The listing builds one solid part. Answer for the finished solid, in the listing's coordinates (mm). A direction names the side the tool comes from. Coordinates: 2 decimals unless noted, no trailing zeros. Loops run counter-clockwise (first coordinate to the right, second up) from the corner with the lowest first, then second, coordinate; pieces in that order, holes last. Notation, with made-up numbers: M 74,-17 L 129,-17 A13 ccw 129,-7 Z; hole C 80,-24 d10. An arc over 180 degrees is marked long. Answer as a JSON object with one key per item and string values. Group by question number.
1. A cutting plane is placed at C-C on x = 0. Give the vertices of the cut face in (y, z).
2. Determine the mould class of faces 5 (the face through (0, -20.32, 19)), 6 (the face through (-38.735, -25, 19)), 7 (the face through (38.011, -21.084, 19.317)) for opening direction X: released by +X, released by -X, zero draft, split by the parting line, or undercut.
3. A cutting plane is placed at A-A on y = 0. Give the vertices of the cut face in (x, z).
4. For faces 1 (the face through (-22.949, -19.556, 19.317)), 2 (the face through (15.875, -16, 19)), 3 (the face through (22.38, -12.44, 19.32)), 4 (the face through (0.132, -24.792, 16.244)), determine the directions among +Z, -Z, +X, -X, +Y, -Y from which every point of the face is accessible in a straight line to the end or side of a thin tool.
5. Given pin 1 (6 mm diameter, centred on x = -31.115, z = 6.35, fed in from +Y); pin 2 (5.5 mm diameter, centred on x = 30.5, z = 19, fed in from +Y); pin 3 (4.5 mm diameter, centred on y = -16, z = 24, fed in from +X); pin 4 (8 mm diameter, centred on y = -15, z = 24, fed in from +X), each flat-ended and moving along its own axis, determine where each tip first touches the part or whether it passes through.
6. Straight lines are drawn through the part: L1, parallel to Z at x = 0, y = -25.65; L2, parallel to X at y = -23, z = 31.75 (3 decimals); L3, parallel to X at y = -22, z = 31.75. For each, find the intervals that lie inside material, in ascending order.
7. A cutting plane is placed at B-B on z = 6.35. State how many separate pieces and enclosed holes the cut face has, and give its area (3 significant figures).
from build123d import *

# Parameters (mm, degrees)
BOSS_EXTRUDE1_DEPTH = 38.1
FILLET1_R           = 6.35
CUT_EXTRUDE1_REACH  = 71.34
SKETCH2_R           = 1.7
SKETCH2_3_R         = 3
SKETCH2_3_R_2       = 1.7
CUT_EXTRUDE2_DEPTH  = 6.35
SKETCH5_W           = 38.1
SKETCH5_H           = 6.35
BOSS_EXTRUDE3_DEPTH = 16.51
SKETCH6_R           = 3.3782
CUT_EXTRUDE3_DEPTH  = 76.254867783
FILLET2_R           = 2.54
BOSS_EXTRUDE4_START = -2.54
SKETCH7_R           = 3
SKETCH7_R_2         = 1.5
BOSS_EXTRUDE4_DEPTH = 2.54


with BuildPart() as part:
    # Sketch1 → Boss-Extrude1 (new body)
    with BuildSketch(Plane.XY):
        with BuildLine():
            Line((22.225, -26.67), (22.225, -12.296722124))
            ThreePointArc((22.225, -12.296722124), (0, 25.4), (-22.225, -12.296722124))
            Line((-22.225, -12.296722124), (-22.225, -26.67))
            Line((-22.225, -26.67), (22.225, -26.67))
        make_face()
        with BuildLine():
            Line((-15.875, -20.32), (15.875, -20.32))
            Line((15.875, -20.32), (15.875, -10.530283709))
            ThreePointArc((15.875, -10.530283709), (0, 19.05), (-15.875, -10.530283709))
            Line((-15.875, -10.530283709), (-15.875, -20.32))
        make_face(mode=Mode.SUBTRACT)
    extrude(amount=BOSS_EXTRUDE1_DEPTH)

    # Fillet1
    fillet1_edges = [part.edges().sort_by_distance(p)[0] for p in [
        (-15.875, -10.530283709, 19.05),
        (15.875, -10.530283709, 19.05),
        (22.225, -12.296722124, 19.05),
        (-22.225, -12.296722124, 19.05),
    ]]
    fillet(fillet1_edges, radius=FILLET1_R)

    # Sketch2 → Cut-Extrude1 (cut, up to next)
    with BuildSketch(Plane.XZ.offset(26.67), mode=Mode.PRIVATE) as cut_extrude1_sk1:
        with Locations(Location((0, 32.2471478, 0), (0, 0, 270))):
            Circle(SKETCH2_R)
    cut_extrude1_tool1 = extrude(cut_extrude1_sk1.sketch, amount=-CUT_EXTRUDE1_REACH, mode=Mode.PRIVATE) & part.part
    # Sketch2 → Cut-Extrude1 (cut, up to next)
    with BuildSketch(Plane.XZ.offset(26.67), mode=Mode.PRIVATE) as cut_extrude1_sk2:
        with Locations(Location((0, 13.2471478, 0), (0, 0, 270))):
            Circle(SKETCH2_R)
    cut_extrude1_tool2 = extrude(cut_extrude1_sk2.sketch, amount=-CUT_EXTRUDE1_REACH, mode=Mode.PRIVATE) & part.part
    add(cut_extrude1_tool1.solids().sort_by_distance((0, -26.67, 32.247148))[0], mode=Mode.SUBTRACT)
    add(cut_extrude1_tool2.solids().sort_by_distance((0, -26.67, 13.247148))[0], mode=Mode.SUBTRACT)

    # Sketch2_3 → Cut-Extrude2 (cut)
    # profile 1 of 2: a face of its own
    with BuildSketch(Plane.XZ.offset(26.67)):
        with Locations(Location((0, 32.2471478, 0), (0, 0, 270))):
            Circle(SKETCH2_3_R)
        with Locations((0, 32.2471478)):
            Circle(SKETCH2_3_R_2, mode=Mode.SUBTRACT)
    # profile 2 of 2: a face of its own
    with BuildSketch(Plane.XZ.offset(26.67)):
        with Locations(Location((0, 13.2471478, 0), (0, 0, 270))):
            Circle(SKETCH2_3_R)
        with Locations((0, 13.2471478)):
            Circle(SKETCH2_3_R_2, mode=Mode.SUBTRACT)
    extrude(amount=-CUT_EXTRUDE2_DEPTH, mode=Mode.SUBTRACT)

    # Sketch5 → Boss-Extrude3 (add)
    with BuildSketch(Plane.ZY.offset(22.225)):
        with Locations((19.05, -23.495)):
            Rectangle(SKETCH5_W, SKETCH5_H)
    boss_extrude3 = extrude(amount=BOSS_EXTRUDE3_DEPTH)

    # Sketch6 → Cut-Extrude3 (cut, through all)
    with BuildSketch(Plane(origin=(0, -26.67, 0), x_dir=(-1, 0, 0), z_dir=(0, -1, 0))):
        with Locations(Location((31.115, -6.35, 0), (0, 0, 90))):
            Circle(SKETCH6_R)
        with Locations(Location((31.115, -31.75, 0), (0, 0, 90))):
            Circle(SKETCH6_R)
    cut_extrude3 = extrude(amount=-CUT_EXTRUDE3_DEPTH, mode=Mode.SUBTRACT)

    # Mirror1: Boss-Extrude3, Cut-Extrude3 across plane
    add(boss_extrude3.mirror(Plane(origin=(0, 0, 0), x_dir=(0, 0, 1), z_dir=(1, 0, 0))))
    add(cut_extrude3.mirror(Plane(origin=(0, 0, 0), x_dir=(0, 0, 1), z_dir=(1, 0, 0))), mode=Mode.SUBTRACT)

    # Fillet2
    fillet2_edges = [part.edges().sort_by_distance(p)[0] for p in [
        (38.735, -20.32, 19.05),
        (22.225, -20.32, 19.05),
        (-22.225, -20.32, 19.05),
        (-38.735, -20.32, 19.05),
    ]]
    fillet(fillet2_edges, radius=FILLET2_R)

    # Sketch7 → Boss-Extrude4 (add)
    # profile 1 of 2: a face of its own
    with BuildSketch(Plane(origin=(0, -20.32, 0), x_dir=(1, 0, 0), z_dir=(0, 1, 0)).offset(BOSS_EXTRUDE4_START)):
        with Locations(Location((0, -13.2471478, 0), (0, 0, 90))):
            Circle(SKETCH7_R)
        with Locations(Location((0, -13.2471478, 0), (0, 0, 270))):
            Circle(SKETCH7_R_2, mode=Mode.SUBTRACT)
    # profile 2 of 2: a face of its own
    with BuildSketch(Plane(origin=(0, -20.32, 0), x_dir=(1, 0, 0), z_dir=(0, 1, 0)).offset(BOSS_EXTRUDE4_START)):
        with Locations(Location((0, -32.2471478, 0), (0, 0, 90))):
            Circle(SKETCH7_R)
        with Locations(Location((0, -32.2471478, 0), (0, 0, 270))):
            Circle(SKETCH7_R_2, mode=Mode.SUBTRACT)
    extrude(amount=BOSS_EXTRUDE4_DEPTH)


solid = part.part
From the geometry:
{
 "1": {"outline": "M -26.67,0 L -20.32,0 L -20.32,11.75 L -22.86,11.75 L -22.86,10.25 L -26.67,10.25 Z; M -26.67,16.25 L -22.86,16.25 L -22.86,14.75 L -20.32,14.75 L -20.32,30.75 L -22.86,30.75 L -22.86,29.25 L -26.67,29.25 Z; M -26.67,35.25 L -22.86,35.25 L -22.86,33.75 L -20.32,33.75 L -20.32,38.1 L -26.67,38.1 Z; M 19.05,0 L 25.4,0 L 25.4,38.1 L 19.05,38.1 Z"},
 "2": {"face 5": "undercut", "face 6": "released by -X", "face 7": "released by +X"},
 "3": {"outline": "M -25.4,0 L -19.05,0 L -19.05,38.1 L -25.4,38.1 Z; M 19.05,0 L 25.4,0 L 25.4,38.1 L 19.05,38.1 Z"},
 "4": {"face 1": "+Z, -Z, -X", "face 2": "+Z, -Z", "face 3": "+Z, -Z, +X", "face 4": "-Y"},
 "5": {"pin 1": "passes through", "pin 2": "stops at y = -20.32", "pin 3": "stops at x = 22.27", "pin 4": "stops at x = 22.89"},
 "6": {"L1": "z = 0 to 10.25, 16.25 to 29.25, 35.25 to 38.1", "L2": "x = -38.735 to -34.493, -27.737 to -2.959, 2.959 to 27.737, 34.493 to 38.735", "L3": "x = -38.58 to -34.49, -27.74 to -1.42, 1.42 to 27.74, 34.49 to 38.58"},
 "7": {"separate pieces": "3", "enclosed holes": "1", "area": "1,110 mm²"}
}
